Model file for the job. Use its own axes, mm. A direction names the side the tool comes from. Round coordinates to 2 decimals unless told otherwise and drop trailing zeros. Loops run counter-clockwise (first coordinate to the right, second up) from the corner with the lowest first, then second, coordinate; pieces in that order, holes last. Notation, with made-up numbers: (42, 78.25) - (48, 78.25) arc R19 ccw to (48, 84.25) - close; hole circle Ø10 at (-32.5, -38). An arc over 180 degrees is marked (long way). Answer as a JSON object with one key per item and string values.
from build123d import *

# Parameters (mm, degrees)
F0_R           = 55
F0_R_2         = 3
F1_DEPTH       = 50
F2_R           = 38.5
F2_R_2         = 3
F3_DEPTH       = 33
F5_D           = 6.6
F5_CBORE_D     = 11.25
F5_CBORE_DEPTH = 6
F6_R           = 57.5
F6_R_2         = 45
F7_DEPTH       = 40


with BuildPart() as f1:
    # F0 (on Top) → F1 (new body)
    with BuildSketch(Plane.XY):
        Circle(F0_R)
        with BuildLine():
            ThreePointArc((28.0281341694, -14.45), (25.8045913047, -17.3477774789), (22.430057958, -15.95))
            Line((22.430057958, -15.95), (2.5980762114, -27.4))
            ThreePointArc((2.5980762114, -27.4), (2.8977774789, -28.1235428647), (3, -28.9))
            ThreePointArc((3, -28.9), (-0.7764571353, -31.7977774789), (-2.5980762114, -27.4))
            Line((-2.5980762114, -27.4), (-22.430057958, -15.95))
            ThreePointArc((-22.430057958, -15.95), (-27.6262103807, -15.95), (-25.0281341694, -11.45))
            Line((-25.0281341694, -11.45), (-25.0281341694, 11.45))
            ThreePointArc((-25.0281341694, 11.45), (-27.6262103807, 15.95), (-22.430057958, 15.95))
            Line((-22.430057958, 15.95), (-2.5980762114, 27.4))
            ThreePointArc((-2.5980762114, 27.4), (-0.7764571353, 31.7977774789), (3, 28.9))
            ThreePointArc((3, 28.9), (2.8977774789, 28.1235428647), (2.5980762114, 27.4))
            Line((2.5980762114, 27.4), (22.430057958, 15.95))
            ThreePointArc((22.430057958, 15.95), (25.8045913047, 17.3477774789), (28.0281341694, 14.45))
            ThreePointArc((28.0281341694, 14.45), (27.1494545129, 12.3286796564), (25.0281341694, 11.45))
            Line((25.0281341694, 11.45), (25.0281341694, -11.45))
            ThreePointArc((25.0281341694, -11.45), (27.1494545129, -12.3286796564), (28.0281341694, -14.45))
        make_face(mode=Mode.SUBTRACT)
        with BuildLine():
            Line((2.5980762114, -27.4), (22.430057958, -15.95))
            ThreePointArc((22.430057958, -15.95), (22.430057958, -12.95), (25.0281341694, -11.45))
            Line((25.0281341694, -11.45), (25.0281341694, 11.45))
            ThreePointArc((25.0281341694, 11.45), (22.430057958, 12.95), (22.430057958, 15.95))
            Line((22.430057958, 15.95), (2.5980762114, 27.4))
            ThreePointArc((2.5980762114, 27.4), (0, 25.9), (-2.5980762114, 27.4))
            Line((-2.5980762114, 27.4), (-22.430057958, 15.95))
            ThreePointArc((-22.430057958, 15.95), (-22.1303566905, 15.2264571353), (-22.0281341694, 14.45))
            ThreePointArc((-22.0281341694, 14.45), (-22.9068138258, 12.3286796564), (-25.0281341694, 11.45))
            Line((-25.0281341694, 11.45), (-25.0281341694, -11.45))
            ThreePointArc((-25.0281341694, -11.45), (-22.9068138258, -12.3286796564), (-22.0281341694, -14.45))
            ThreePointArc((-22.0281341694, -14.45), (-22.1303566905, -15.2264571353), (-22.430057958, -15.95))
            Line((-22.430057958, -15.95), (-2.5980762114, -27.4))
            ThreePointArc((-2.5980762114, -27.4), (0, -25.9), (2.5980762114, -27.4))
        make_face()
        Circle(F0_R_2, mode=Mode.SUBTRACT)
    extrude(amount=F1_DEPTH)

    # F2 (on face) → F3 (cut)
    with BuildSketch(Plane.XY.offset(50)):
        Circle(F2_R)
        with Locations((-25.0281341694, -14.45)):
            Circle(F2_R_2, mode=Mode.SUBTRACT)
        with Locations((0, -28.9)):
            Circle(F2_R_2, mode=Mode.SUBTRACT)
        with Locations((25.0281341694, -14.45)):
            Circle(F2_R_2, mode=Mode.SUBTRACT)
        with Locations((-25.0281341694, 14.45)):
            Circle(F2_R_2, mode=Mode.SUBTRACT)
        Circle(F2_R_2, mode=Mode.SUBTRACT)
        with Locations((25.0281341694, 14.45)):
            Circle(F2_R_2, mode=Mode.SUBTRACT)
        with Locations((0, 28.9)):
            Circle(F2_R_2, mode=Mode.SUBTRACT)
    extrude(amount=-F3_DEPTH, mode=Mode.SUBTRACT)

    # F5 (through all)
    with Locations(Plane.XY.offset(17)):
        with Locations((-25.0281341694, 14.45), (-25.0281341694, -14.45), (0, -28.9), (25.0281341694, -14.45), (25.0281341694, 14.45), (0, 28.9), (0, 0)):
            CounterBoreHole(F5_D / 2, F5_CBORE_D / 2, F5_CBORE_DEPTH)

    # F6 (on face) → F7 (cut)
    with BuildSketch(Plane(origin=(0, 0, 0), x_dir=(1, 0, 0), z_dir=(0, 0, -1))):
        Circle(F6_R)
        Circle(F6_R_2, mode=Mode.SUBTRACT)
    extrude(amount=-F7_DEPTH, mode=Mode.SUBTRACT)


solid = f1.part
1) Slice it at C-C on x = 26. List the corners of the cut face in (y, z).
Values follow:
{"outline": "(-48.47, 40) - (-36.73, 40) - (-36.73, 0) - (-17.6, 0) - (-17.6, 11) - (-19.99, 11) - (-19.99, 17) - (-28.39, 17) - (-28.39, 50) - (-48.47, 50) - close; (-11.3, 0) - (11.3, 0) - (11.3, 11) - (8.91, 11) - (8.91, 17) - (-8.91, 17) - (-8.91, 11) - (-11.3, 11) - close; (17.6, 0) - (36.73, 0) - (36.73, 40) - (48.47, 40) - (48.47, 50) - (28.39, 50) - (28.39, 17) - (19.99, 17) - (19.99, 11) - (17.6, 11) - close"}
2) Slice it at D-D on y = 14.45. List the corners of the cut face in (x, z).
Values follow:
{"outline": "(-53.07, 40) - (-42.62, 40) - (-42.62, 0) - (-28.33, 0) - (-28.33, 11) - (-30.65, 11) - (-30.65, 17) - (-35.69, 17) - (-35.69, 50) - (-53.07, 50) - close; (-21.73, 0) - (21.73, 0) - (21.73, 11) - (19.4, 11) - (19.4, 17) - (-19.4, 17) - (-19.4, 11) - (-21.73, 11) - close; (28.33, 0) - (42.62, 0) - (42.62, 40) - (53.07, 40) - (53.07, 50) - (35.69, 50) - (35.69, 17) - (30.65, 17) - (30.65, 11) - (28.33, 11) - close"}
3) Tool access for faces 4 (the flat face through (11.5, 37.4, 50)), 5 (the cylindrical face through (-19.83, 12.3, 14.04)): list every direction of +Z, -Z, +X, -X, +Y, -Y with a clear straight run to the whole face (end or side of a thin tool).
Values follow:
{"face 4": "+Z, +X, -X, +Y, -Y", "face 5": "+Z"}
4) Two-plate mould, pull along X, no slides. Class faces 1 (the flat face through (-21, 40, 40)), 2 (the cylindrical face through (-11.923, -53.692, 44.93)), 3 (the flat face through (0, -4, 11)): pulls with the +X half, pulls with the -X half, needs draft (parallel to the pull), parting line crosses it, or undercut.
Values follow:
{"face 1": "needs draft", "face 2": "parting line crosses it", "face 3": "undercut"}
5) Probe probe 1 along Y at (x, z) = (24, 11.5); probe 2 along Y at (x, z) = (-1, 36); probe 3 along Y at (x, z) = (24, 9.5). List the from-to ranges inside material, lowest first.
Values follow:
{"probe 1": "-38.07 to -19.98, -8.92 to 8.92, 19.98 to 38.07", "probe 2": "-44.99 to -38.49, 38.49 to 44.99", "probe 3": "-38.07 to -17.59, -11.31 to 11.31, 17.59 to 38.07"}
6) Slice it at B-B on z = 8.5. List the corners of the cut face in (x, y), then the cut area to 3 significant figures.
Values follow:
{"outline": "circle Ø90 at (0, 0); hole circle Ø6.6 at (-25.03, -14.45); hole circle Ø6.6 at (-25.03, 14.45); hole circle Ø6.6 at (0, -28.9); hole circle Ø6.6 at (0, 0); hole circle Ø6.6 at (0, 28.9); hole circle Ø6.6 at (25.03, -14.45); hole circle Ø6.6 at (25.03, 14.45)", "area": "6,120 mm²"}
7) Slice it at A-A on y = 0. List the corners of the cut face in (x, z) (3 decimals).
Values follow:
{"outline": "(-55, 40) - (-45, 40) - (-45, 0) - (-3.3, 0) - (-3.3, 11) - (-5.625, 11) - (-5.625, 17) - (-38.5, 17) - (-38.5, 50) - (-55, 50) - close; (3.3, 0) - (45, 0) - (45, 40) - (55, 40) - (55, 50) - (38.5, 50) - (38.5, 17) - (5.625, 17) - (5.625, 11) - (3.3, 11) - close"}
8) Drop flat-ended pins along their axis: P1, Ø4, axis at x = -10.5, z = 23, coming from the +Y side; P2, Ø1.5, axis at y = -22.5, z = 17.5, coming from the +X side; P3, Ø4, axis at x = 0, y = 28.9, coming from the +Z side; P4, Ø6, axis at y = -24, z = 20, coming from the -X side. Give the stop position or say it passes through.
Values follow:
{"P1": "y = 44.19", "P2": "x = 39.39", "P3": "through", "P4": "x = -39.8"}
